from build123d import *

# Parameters (mm, degrees)
SKETCH1_W           = 120
SKETCH1_H           = 100
BOSS_EXTRUDE1_DEPTH = 5
SKETCH2_R           = 2.5
CUT_EXTRUDE1_DEPTH  = 6
SKETCH3_W           = 120
SKETCH3_H           = 2
BOSS_EXTRUDE2_DEPTH = 20
CUT_EXTRUDE2_DEPTH  = 26
CUT_EXTRUDE3_DEPTH  = 26
SKETCH6_W           = 5
SKETCH6_H           = 30
BOSS_EXTRUDE3_DEPTH = 20
CUT_EXTRUDE4_DEPTH  = 106


with BuildPart() as part:
    # Sketch1 → Boss-Extrude1 (new body)
    with BuildSketch(Plane.XY):
        with Locations((60, 50)):
            Rectangle(SKETCH1_W, SKETCH1_H)
    extrude(amount=BOSS_EXTRUDE1_DEPTH)

    # Sketch2 → Cut-Extrude1 (cut, through all)
    with BuildSketch(Plane.XY.offset(5)):
        with Locations((48.561388608, 53.909722104)):
            Circle(SKETCH2_R)
        with BuildLine():
            ThreePointArc((82.975974789, 4.760599446), (92.719162031, 13.288409394), (100.405906554, 23.707967867))
            ThreePointArc((100.405906554, 23.707967867), (95.896997447, 40.800941239), (78.804024076, 36.292032133))
            ThreePointArc((78.804024076, 36.292032133), (74.320089771, 30.213956356), (68.63656388, 25.239400554))
            ThreePointArc((68.63656388, 25.239400554), (65.566868781, 7.830294546), (82.975974789, 4.760599446))
        make_face()
    extrude(amount=-CUT_EXTRUDE1_DEPTH, mode=Mode.SUBTRACT)

    # Sketch3 → Boss-Extrude2 (add)
    with BuildSketch(Plane(origin=(0, 0, 0), x_dir=(-1, 0, 0), z_dir=(0, 0, -1))):
        with Locations((-60, 1)):
            Rectangle(SKETCH3_W, SKETCH3_H)
    extrude(amount=BOSS_EXTRUDE2_DEPTH)

    # Sketch4 → Cut-Extrude2 (cut, through all)
    with BuildSketch(Plane.XY.offset(5)):
        with BuildLine():
            ThreePointArc((66.494283868, 35.596794606), (72.644903394, 39.60143936), (75.487572744, 46.368013909))
            ThreePointArc((75.487572744, 46.368013909), (73.248961533, 49.104548186), (70.512427256, 46.865936976))
            ThreePointArc((70.512427256, 46.865936976), (68.806825647, 42.805992246), (65.116453931, 40.403205394))
            ThreePointArc((65.116453931, 40.403205394), (63.402163505, 37.311085032), (66.494283868, 35.596794606))
        make_face()
    extrude(amount=-CUT_EXTRUDE2_DEPTH, mode=Mode.SUBTRACT)

    # Sketch5 → Cut-Extrude3 (cut, through all)
    with BuildSketch(Plane.XY.offset(5)):
        with BuildLine():
            Line((120, 70), (48.561388608, 70))
            ThreePointArc((48.561388608, 70), (39.016134462, 66.862913451), (33.192915272, 58.674915711))
            Line((33.192915272, 58.674915711), (15, 0))
            Line((15, 0), (0, 0))
            Line((0, 0), (0, 100))
            Line((0, 100), (120, 100))
            Line((120, 100), (120, 70))
        make_face()
    extrude(amount=-CUT_EXTRUDE3_DEPTH, mode=Mode.SUBTRACT)

    # Sketch6 → Boss-Extrude3 (add, through all)
    with BuildSketch(Plane(origin=(0, 0, 0), x_dir=(-1, 0, 0), z_dir=(0, 0, -1))):
        with Locations((-117.5, 15)):
            Rectangle(SKETCH6_W, SKETCH6_H)
        with Locations((-32.5, 15)):
            Rectangle(SKETCH6_W, SKETCH6_H)
    extrude(amount=BOSS_EXTRUDE3_DEPTH)

    # Sketch9 → Cut-Extrude4 (cut, through all)
    with BuildSketch(Plane(origin=(120, 0, 0), x_dir=(0, 0, -1), z_dir=(1, 0, 0))):
        Polygon((0, 30), (20, 0), (20, 30), align=None)
    extrude(amount=-CUT_EXTRUDE4_DEPTH, mode=Mode.SUBTRACT)


solid = part.part
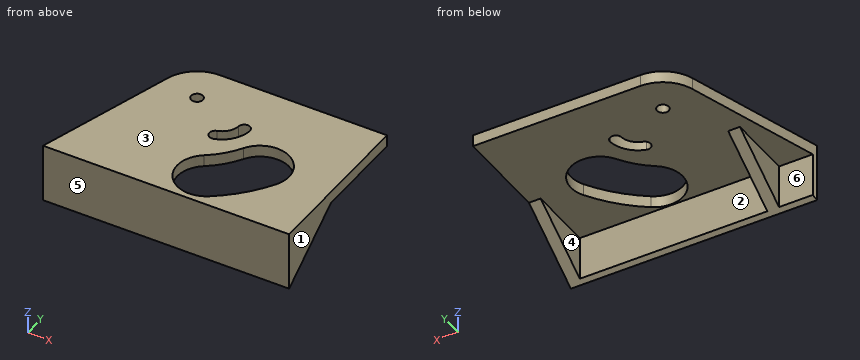
CAD build for the part. Positions are in the model's coordinates, mm. Face numbers are marked on the shaded views. A direction names the side the tool comes from. Coordinates: 2 decimals unless noted, no trailing zeros. Loops run counter-clockwise (first coordinate to the right, second up) from the corner with the lowest first, then second, coordinate; pieces in that order, holes last. Notation, with made-up numbers: (42.5, 20.25) - (91.5, 20.25) arc R15 cw to (91.5, 25.25) - close; hole circle Ø10 at (-16.5, 35). An arc over 180 degrees is marked (long way). Write item = value, one per line. Start each with the question number.
Q1. Cut at D-D, the plane z = 2.5. List the corners of the cut face in (x, y).
Q2. Cut at B-B, the plane y = 34. List the corners of the cut face in (x, z), then the cut area to 3 significant figures.
Q3. Cut at A-A, the plane z = -13. List the corners of the cut face in (x, y), then the cut area to 3 significant figures.
Q4. Pull direction X, two halves, no side cores. Call the marked faces 1, 2 and 3: pulls with the +X half, pulls with the -X half, needs draft (parallel to the pull), parting line crosses it, or undercut.
Q5. Cut at C-C, the plane x = 111. List the corners of the cut face in (y, z), then the cut area to 3 significant figures.
Q6. Flat gauge pins, fed straight in: pin 1 Ø3 at (x, z) = (83.5, -17) entering from +Y; pin 2 Ø4 at (x, y) = (48.56, 53.91) entering from +Z; pin 3 Ø9.5 at (y, z) = (14.5, -11) entering from -X; pin 4 Ø5 at (x, y) = (38.5, 30) entering from -Z. Where does each tip first touch, or does it go through?
Q7. Which spindle directions (+Z, -Z, +X, -X, +Y, -Y) get a long thin tool onto all of the face, cutting with end or side? Do the marked faces 4, 5 and 6. Say none if no direction does.
Q8. Drill centre lines: L1, parallel to X at y = 8, z = -1.75; L2, parallel to Z at x = 109.5, y = 46; L3, parallel to Y at x = 72.5, z = -14.5. Where is each one in solid material? Low to high.
Computed:
q1.outline = (15, 0) - (120, 0) - (120, 70) - (48.56, 70) arc R16.09 ccw to (33.19, 58.67) - close; hole circle Ø5 at (48.56, 53.91); hole (65.12, 40.4) arc R2.5 ccw to (66.49, 35.6) arc R12.5 ccw to (75.49, 46.37) arc R2.5 ccw to (70.51, 46.87) arc R7.5 cw to start; hole (68.64, 25.24) arc R12.5 ccw to (82.98, 4.76) arc R60 ccw to (100.41, 23.71) arc R12.5 ccw to (78.8, 36.29) arc R35 cw to start
q2.outline = (25.54, 0) - (77.35, 0) - (77.35, 5) - (25.54, 5) - close; (101.45, 0) - (120, 0) - (120, 5) - (101.45, 5) - close
q2.area = 352 mm²
q3.outline = (15, 0) - (120, 0) - (120, 10.5) - (115, 10.5) - (115, 2) - (35, 2) - (35, 10.5) - (30, 10.5) - (30, 2) - (15.62, 2) - close
q3.area = 294 mm²
q4.face_1 = pulls with the +X half
q4.face_2 = undercut
q4.face_3 = needs draft
q5.outline = (0, -20) - (2, -18.67) - (2, 0) - (70, 0) - (70, 5) - (0, 5) - close
q5.area = 389 mm²
q6.pin_1 = 2
q6.pin_2 = through
q6.pin_3 = 30
q6.pin_4 = 0
q7.face_4 = -Z, +Y
q7.face_5 = +Z, -Z, +X, -X, -Y
q7.face_6 = -Z, -X, +Y
q8.L1 = 30 to 35, 115 to 120
q8.L2 = 0 to 5
q8.L3 = 0 to 2
